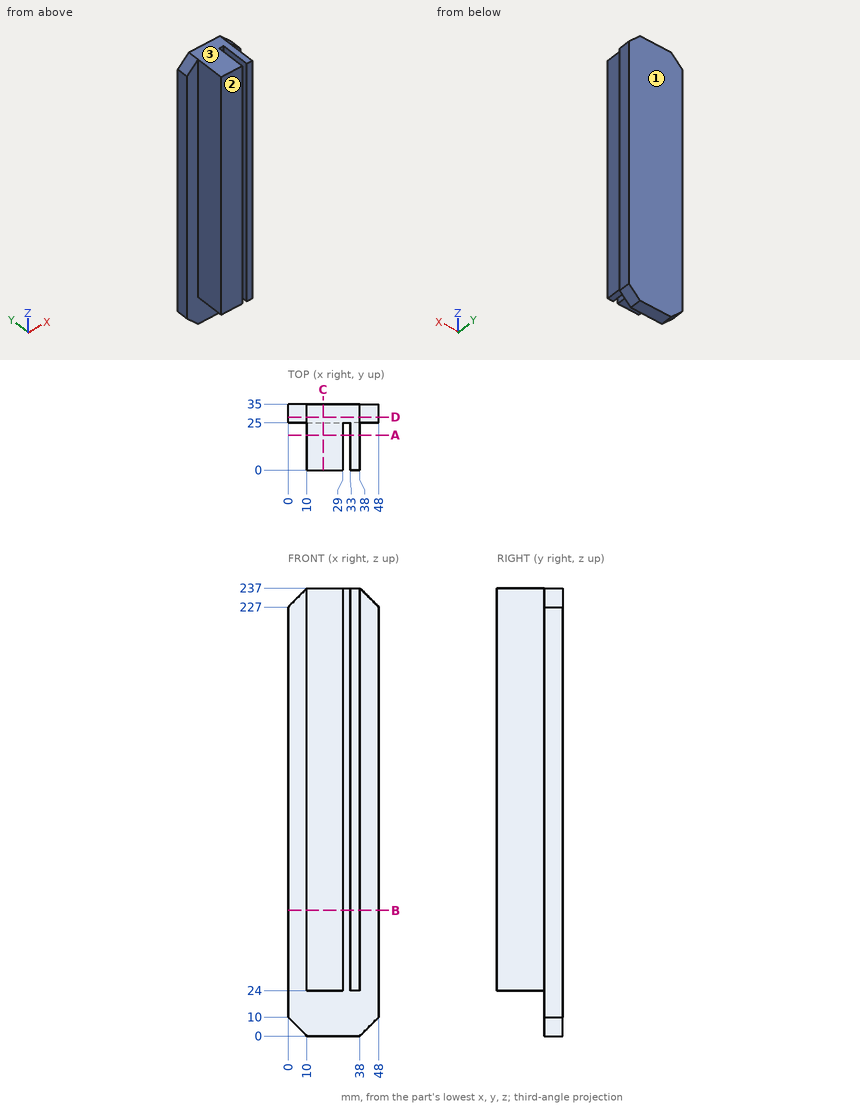
Source: three-view drawing plus pictorial views. Frame: mm from the lowest corner of the part. Coordinates: 2 decimals unless noted, no trailing zeros. Order: outer loops, then holes, each group sorted by start corner. A loop starts at its lowest first (then second) coordinate and runs counter-clockwise, first axis right, second up. Notation, with made-up numbers: M 30.5,-12 L 88.5,-12 A16 cw 88.5,-2 Z; hole C -22,63 d5. An arc over 180 degrees is marked long. Write each question's results on one line, items separated by ' | '. Start each with the question number.
1. Section C-C, the plane x = 18.5. Return the cut outline in (y, z).
2. Pin query (flat end, axial travel): pin 1 (7.5 mm diameter, centred on y = 16, z = 158, fed in from +X); pin 2 (4 mm diameter, centred on y = 7.5, z = 29, fed in from -X); pin 3 (4 mm diameter, centred on x = 36, y = 11, fed in from -Z). Return the tip coordinate at first contact, or that it passes through.
3. Draft query along Y for the marked faces 1, 2 and 3. Return one class per face: +Y half, -Y half, draft (parallel to the pull), parting line (faces both ways), or undercut.
4. Section A-A, the plane y = 18.5. Return the cut outline in (x, z), then the cut area to 3 significant figures.
5. Section D-D, the plane y = 28. Return the cut outline in (x, z).
6. Material intervals for L1, parallel to X at y = 19, z = 103; L2, parallel to Z at x = 20, y = 7; L3, parallel to Y at x = 39, z = 30, sorted ascending.
7. Section B-B, the plane z = 66.5. Return the cut outline in (x, y), then the cut area to 3 significant figures.
Solution:
1) outline: M 0,24 L 25,24 L 25,0 L 35,0 L 35,237 L 0,237 Z
2) pin 1: x = 38 | pin 2: x = 10 | pin 3: z = 24
3) face 1: +Y half | face 2: -Y half | face 3: draft
4) outline: M 10,24 L 29,24 L 29,237 L 10,237 Z; M 33,24 L 38,24 L 38,237 L 33,237 Z | area: 5,110 mm²
5) outline: M 0,10 L 10,0 L 38,0 L 48,10 L 48,227 L 38,237 L 10,237 L 0,227 Z
6) L1: 10 to 29, 33 to 38 | L2: 24 to 237 | L3: 25 to 35
7) outline: M 0,25 L 10,25 L 10,0 L 29,0 L 29,25 L 33,25 L 33,0 L 38,0 L 38,25 L 48,25 L 48,35 L 0,35 Z | area: 1,080 mm²
